Input: part model. Units: mm. Frame: model coordinates. Coordinates: 2 decimals unless noted, no trailing zeros. Write each loop counter-clockwise with the first axis right and the second up, starting at its lowest first coordinate (ties: lowest second). Pieces come first, ordered by that corner, then holes. Notation, with made-up numbers: (21, 29.5) - (33, 29.5) arc R23 cw to (33, 60.5) - close; hole circle Ø1 at (85, -15.5). An arc over 180 degrees is marked (long way). Use a Markdown table: item, result. Add a question column.
Q1. Pin query (flat end, axial travel): P1, Ø4, axis at x = -1, z = -8.5, coming from the -Y side; P2, Ø15, axis at x = -55.75, z = 0, coming from the +Y side; P3, Ø10, axis at y = -12, z = -14.5, coming from the +X side; P4, Ø1, axis at x = -30, y = -5.5, coming from the +Z side. Return the tip coordinate at first contact, or that it passes through.
Q2. Section query B-B (y = -18). Return the cut outline in (x, z).
Q3. Mould query, pull axis X, two halves, no side actions, for faces 1 (the face through (76.197, -6.261, -0.343)), 2 (the face through (-43.63, -6.26, 3.81)), 3 (the face through (56, -20.32, 0)). Classes: released by +X, released by -X, zero draft, split by the parting line, or undercut.
Q4. Material intervals for probe 1 along X at (y, z) = (-11.75, 0.5); probe 2 along X at (y, z) = (-11, 2); probe 3 along Y at (x, z) = (35.5, -1.5), sorted ascending. Write a range as from..to.
from build123d import *

# Parameters (mm, degrees)
F0_R     = 12.7
F0_R_2   = 16.51
F1_DEPTH = 12.7
F2_DEPTH = 20.32
F3_R     = 7.61999


# Not quite as in the source:
# - a fillet or chamfer is up to 0.001 mm smaller than in the source, because OpenCascade refuses the exact size


with BuildPart() as f1:
    # F0 (on Front) → F1 (new body)
    with BuildSketch(Plane.XZ):
        with BuildLine():
            add(Edge.make_bspline(
                [(63.1930127424, -19.05), (57.8929819167, -20.9148749709), (49.1822585518, -19.6780685204), (34.4123652883, -13.7010865969), (20.7204562035, -10.3509186108), (5.798157397, -8.9775289718), (1.5977957695, -9.0970061045), (0, -9.1456407681)],
                knots=[0, 0, 0, 0, 0.2119684652, 0.4335943825, 0.6511337867, 0.8674060842, 1, 1, 1, 1], degree=3))
            ThreePointArc((63.1930127424, -19.05), (76.2, 0), (63.1930127424, 19.05))
            add(Edge.make_bspline(
                [(63.1930127424, 19.05), (57.8929819167, 20.9148749709), (49.1822585518, 19.6780685204), (34.4123652883, 13.7010865969), (20.7204562035, 10.3509186108), (5.798157397, 8.9775289718), (1.5977957695, 9.0970061045), (0, 9.1456407681)],
                knots=[0, 0, 0, 0, 0.2119684652, 0.4335943825, 0.6511337867, 0.8674060842, 1, 1, 1, 1], degree=3))
            add(Edge.make_bspline(
                [(-63.1930127424, 19.05), (-57.8929819167, 20.9148749709), (-49.1822585518, 19.6780685204), (-34.4123652883, 13.7010865969), (-20.7204562035, 10.3509186108), (-5.798157397, 8.9775289718), (-1.5977957695, 9.0970061045), (0, 9.1456407681)],
                knots=[0, 0, 0, 0, 0.2119684652, 0.4335943825, 0.6511337867, 0.8674060842, 1, 1, 1, 1], degree=3))
            ThreePointArc((-63.1930127424, 19.05), (-76.2, 0), (-63.1930127424, -19.05))
            add(Edge.make_bspline(
                [(-63.1930127424, -19.05), (-57.8929819167, -20.9148749709), (-49.1822585518, -19.6780685204), (-34.4123652883, -13.7010865969), (-20.7204562035, -10.3509186108), (-5.798157397, -8.9775289718), (-1.5977957695, -9.0970061045), (0, -9.1456407681)],
                knots=[0, 0, 0, 0, 0.2119684652, 0.4335943825, 0.6511337867, 0.8674060842, 1, 1, 1, 1], degree=3))
        make_face()
        with Locations((-55.7462159306, 0)):
            Circle(F0_R, mode=Mode.SUBTRACT)
        with Locations((55.7462159306, 0)):
            Circle(F0_R_2, mode=Mode.SUBTRACT)
    extrude(amount=F1_DEPTH)

    # F0 (on Front) → F2 (join)
    with BuildSketch(Plane.XZ):
        with Locations((55.7462159306, 0)):
            Circle(F0_R_2)
    extrude(amount=F2_DEPTH)

    # F3 (radius 7.62 in the source; OpenCascade refuses exactly that, so slightly less here)
    f3_edges = [f1.edges().sort_by_distance(p)[0] for p in [
        (39.236216, -20.32, 0),
    ]]
    fillet(f3_edges, radius=F3_R)


solid = f1.part
Values follow:
| question | item | result |
|---|---|---|
| 1 | P1 | y = -12.7 |
| 1 | P2 | through |
| 1 | P3 | x = 73.86 |
| 1 | P4 | z = 12.9 |
| 2 | outline | circle Ø28.73 at (55.75, 0) |
| 3 | face 1 | released by +X |
| 3 | face 2 | undercut |
| 3 | face 3 | zero draft |
| 4 | probe 1 | -76.19..-68.44, -43.06..76.19 |
| 4 | probe 2 | -76.1..-68.29, -43.2..76.1 |
| 4 | probe 3 | -12.7..0 |
